Part model, mm, in its own coordinate system. A direction names the side the tool comes from. Give positions to 0.01 mm unless a question says otherwise; leave off trailing zeros. Order: outer loops, then holes, each group sorted by start corner. A loop starts at its lowest first (then second) coordinate and runs counter-clockwise, first axis right, second up. Notation, with made-up numbers: M 8.5,16 L 62.5,16 A17 ccw 62.5,38 Z; hole C -9.75,-7 d11. An arc over 180 degrees is marked long. Write each question's results on one line, items separated by ' | '. Start each with the question number.
from build123d import *

# Parameters (mm, degrees)
BOSS_EXTRUDE1_DEPTH        = 3
BOSS_EXTRUDE2_DEPTH        = 1.5
BOSS_EXTRUDE2_DEPTH_BACK   = 1.5
SKETCH2_W                  = 37.6
SKETCH2_H                  = 50.8
FILLET2_R                  = 2
CUT_EXTRUDE2_REACH         = 69.217
SKETCH4_R                  = 1.6
CIRPATTERN1_COUNT          = 6
SZKIC1_R                   = 2.5
WYTNIJ_WYCI_GNI_CIE1_DEPTH = 10


with BuildPart() as part:
    # Sketch1 → Boss-Extrude1 (new body)
    with BuildSketch(Plane.XY):
        Polygon((-18.8, 0), (18.8, 0), (18.8, 22), (18.8, 39.799804834), (-18.8, 39.799804834), (-18.8, 22), align=None)
        with BuildLine():
            Line((-6.6, 13.799434154), (-6.6, 27.699434154))
            ThreePointArc((-6.6, 27.699434154), (0, 34.299458505), (6.6, 27.699434154))
            Line((6.6, 27.699434154), (6.6, 13.799434154))
            ThreePointArc((6.6, 13.799434154), (0, 7.199458505), (-6.6, 13.799434154))
        make_face(mode=Mode.SUBTRACT)
    extrude(amount=BOSS_EXTRUDE1_DEPTH)

    # Sketch2 → Boss-Extrude2 (add, two sides: drawn at the far end of the back side and taken through both)
    with BuildSketch(Plane.XZ.offset(-BOSS_EXTRUDE2_DEPTH_BACK)):
        with Locations((0, -22.4)):
            Rectangle(SKETCH2_W, SKETCH2_H)
    extrude(amount=BOSS_EXTRUDE2_DEPTH + BOSS_EXTRUDE2_DEPTH_BACK)

    # Fillet2
    fillet2_edges = [part.edges().sort_by_distance(p)[0] for p in [
        (-18.8, 39.799804834, 1.5),
        (18.8, 39.799804834, 1.5),
        (-18.8, 0, -47.8),
        (18.8, 0, -47.8),
    ]]
    fillet(fillet2_edges, radius=FILLET2_R)

    # Sketch4 → Cut-Extrude2 (cut, up to next)
    with BuildSketch(Plane.XY.offset(3), mode=Mode.PRIVATE) as cut_extrude2_sk1:
        with Locations((7.619805215, 33.947348281)):
            Circle(SKETCH4_R)
    cut_extrude2_tool1 = extrude(cut_extrude2_sk1.sketch, amount=-CUT_EXTRUDE2_REACH, mode=Mode.PRIVATE) & part.part
    # Sketch4 → Cut-Extrude2 (cut, up to next)
    with BuildSketch(Plane.XY.offset(3), mode=Mode.PRIVATE) as cut_extrude2_sk2:
        with Locations((15.23961043, 20.749458505)):
            Circle(SKETCH4_R)
    cut_extrude2_tool2 = extrude(cut_extrude2_sk2.sketch, amount=-CUT_EXTRUDE2_REACH, mode=Mode.PRIVATE) & part.part
    # Sketch4 → Cut-Extrude2 (cut, up to next)
    with BuildSketch(Plane.XY.offset(3), mode=Mode.PRIVATE) as cut_extrude2_sk3:
        with Locations((7.619805215, 7.551568728)):
            Circle(SKETCH4_R)
    cut_extrude2_tool3 = extrude(cut_extrude2_sk3.sketch, amount=-CUT_EXTRUDE2_REACH, mode=Mode.PRIVATE) & part.part
    # Sketch4 → Cut-Extrude2 (cut, up to next)
    with BuildSketch(Plane.XY.offset(3), mode=Mode.PRIVATE) as cut_extrude2_sk4:
        with Locations((-7.619805215, 7.551568728)):
            Circle(SKETCH4_R)
    cut_extrude2_tool4 = extrude(cut_extrude2_sk4.sketch, amount=-CUT_EXTRUDE2_REACH, mode=Mode.PRIVATE) & part.part
    # Sketch4 → Cut-Extrude2 (cut, up to next)
    with BuildSketch(Plane.XY.offset(3), mode=Mode.PRIVATE) as cut_extrude2_sk5:
        with Locations((-15.23961043, 20.749458505)):
            Circle(SKETCH4_R)
    cut_extrude2_tool5 = extrude(cut_extrude2_sk5.sketch, amount=-CUT_EXTRUDE2_REACH, mode=Mode.PRIVATE) & part.part
    # Sketch4 → Cut-Extrude2 (cut, up to next)
    with BuildSketch(Plane.XY.offset(3), mode=Mode.PRIVATE) as cut_extrude2_sk6:
        with Locations((-7.619805215, 33.947348281)):
            Circle(SKETCH4_R)
    cut_extrude2_tool6 = extrude(cut_extrude2_sk6.sketch, amount=-CUT_EXTRUDE2_REACH, mode=Mode.PRIVATE) & part.part
    cut_extrude2_1 = cut_extrude2_tool1.solids().sort_by_distance((7.619805, 33.947348, 3))[0]
    add(cut_extrude2_1, mode=Mode.SUBTRACT)
    cut_extrude2_2 = cut_extrude2_tool2.solids().sort_by_distance((15.23961, 20.749459, 3))[0]
    add(cut_extrude2_2, mode=Mode.SUBTRACT)
    cut_extrude2_3 = cut_extrude2_tool3.solids().sort_by_distance((7.619805, 7.551569, 3))[0]
    add(cut_extrude2_3, mode=Mode.SUBTRACT)
    cut_extrude2_4 = cut_extrude2_tool4.solids().sort_by_distance((-7.619805, 7.551569, 3))[0]
    add(cut_extrude2_4, mode=Mode.SUBTRACT)
    cut_extrude2_5 = cut_extrude2_tool5.solids().sort_by_distance((-15.23961, 20.749459, 3))[0]
    add(cut_extrude2_5, mode=Mode.SUBTRACT)
    cut_extrude2_6 = cut_extrude2_tool6.solids().sort_by_distance((-7.619805, 33.947348, 3))[0]
    add(cut_extrude2_6, mode=Mode.SUBTRACT)
    cut_extrude2 = cut_extrude2_1 + cut_extrude2_2 + cut_extrude2_3 + cut_extrude2_4 + cut_extrude2_5 + cut_extrude2_6  # Cut-Extrude2 as one shape, for the pattern or mirror that repeats it

    # CirPattern1: Cut-Extrude2 ×6 about axis
    cirpattern1_axis = Axis((0, 20.759090909, 0), (0, 0, 1))
    for i in range(1, CIRPATTERN1_COUNT):
        add(cut_extrude2.rotate(cirpattern1_axis, i * 360 / CIRPATTERN1_COUNT), mode=Mode.SUBTRACT)

    # Szkic1 → Wytnij-wyciągnięcie1 (cut)
    with BuildSketch(Plane(origin=(0, 1.5, 0), x_dir=(1, 0, 0), z_dir=(0, 1, 0))):
        with Locations(Location((0, 15, 0), (0, 0, 180))):
            Circle(SZKIC1_R)
        with Locations(Location((0, 35, 0), (0, 0, 180))):
            Circle(SZKIC1_R)
    extrude(amount=-WYTNIJ_WYCI_GNI_CIE1_DEPTH, mode=Mode.SUBTRACT)


solid = part.part
(1) Saw through at C-C on y = 21.5. Give the cut face in (x, z), plus the area to 3 significant figures.
(2) Probe L1, parallel to Z at x = 0, y = 0.85; L2, parallel to Y at x = 9, z = -5; L3, parallel to Z at x = 15, y = 19. List the from-to ranges inside material, lowest first.
(3) Saw through at D-D on x = 10. Give the cut face in (y, z).
(4) Tool access for faces 1 (the cylindrical face through (16.6, 19.9, 1.5)), 2 (the cylindrical face through (18.23, -0.02, -47.2)): list every direction of +Z, -Z, +X, -X, +Y, -Y with a clear straight run to the whole face (end or side of a thin tool).
(5) Drop flat-ended pins along their axis: P1, Ø1.5, axis at x = -0.5, z = -19.5, coming from the +Y side; P2, Ø10, axis at x = -6, y = 18, coming from the -Z side. Give the stop position or say it passes through.
(6) Saw through at A-A on z = -35. Give the cut face in (x, y).
(7) Pull direction X, two halves, no side cores. Call faces 3 (the flat face through (-9, 21, 0)), 4 (the cylindrical face through (-15.23, 22.37, 1.52)), 5 (the cylindrical face through (-18.23, 39.2, 1.52)): +X half, -X half, draft (parallel to the pull), parting line (faces both ways), or undercut.
(8) Saw through at B-B on x = 0. Give the cut face in (y, z).
Taken from the geometry:
1) outline: M -18.8,0 L -16.67,0 L -16.67,3 L -18.8,3 Z; M -13.81,0 L -6.6,0 L -6.6,3 L -13.81,3 Z; M 6.6,0 L 13.81,0 L 13.81,3 L 6.6,3 Z; M 16.67,0 L 18.8,0 L 18.8,3 L 16.67,3 Z | area: 56.1 mm²
2) L1: z = -47.8 to -37.5, -32.5 to -17.5, -12.5 to 3 | L2: y = -1.5 to 1.5 | L3: z = 0 to 3
3) outline: M -1.5,-47.8 L 1.5,-47.8 L 1.5,0 L 39.8,0 L 39.8,3 L -1.5,3 Z
4) face 1: +Z, -Z | face 2: -Z, +X, +Y, -Y
5) P1: stops at y = 1.5 | P2: stops at z = 0
6) outline: M -18.8,-1.5 L -2.5,-1.5 L -2.5,1.5 L -18.8,1.5 Z; M 2.5,-1.5 L 18.8,-1.5 L 18.8,1.5 L 2.5,1.5 Z
7) face 3: draft | face 4: undercut | face 5: -X half
8) outline: M -1.5,-47.8 L 1.5,-47.8 L 1.5,-37.5 L -1.5,-37.5 Z; M -1.5,-32.5 L 1.5,-32.5 L 1.5,-17.5 L -1.5,-17.5 Z; M -1.5,-12.5 L 1.5,-12.5 L 1.5,0 L 7.2,0 L 7.2,3 L -1.5,3 Z; M 34.3,0 L 39.8,0 L 39.8,3 L 34.3,3 Z
